Here's the drawing with two shaded views (mm, measured from the low corner). I have some questions. Coordinates: 2 decimals unless noted, no trailing zeros. Loops run counter-clockwise (first coordinate to the right, second up) from the corner with the lowest first, then second, coordinate; pieces in that order, holes last.
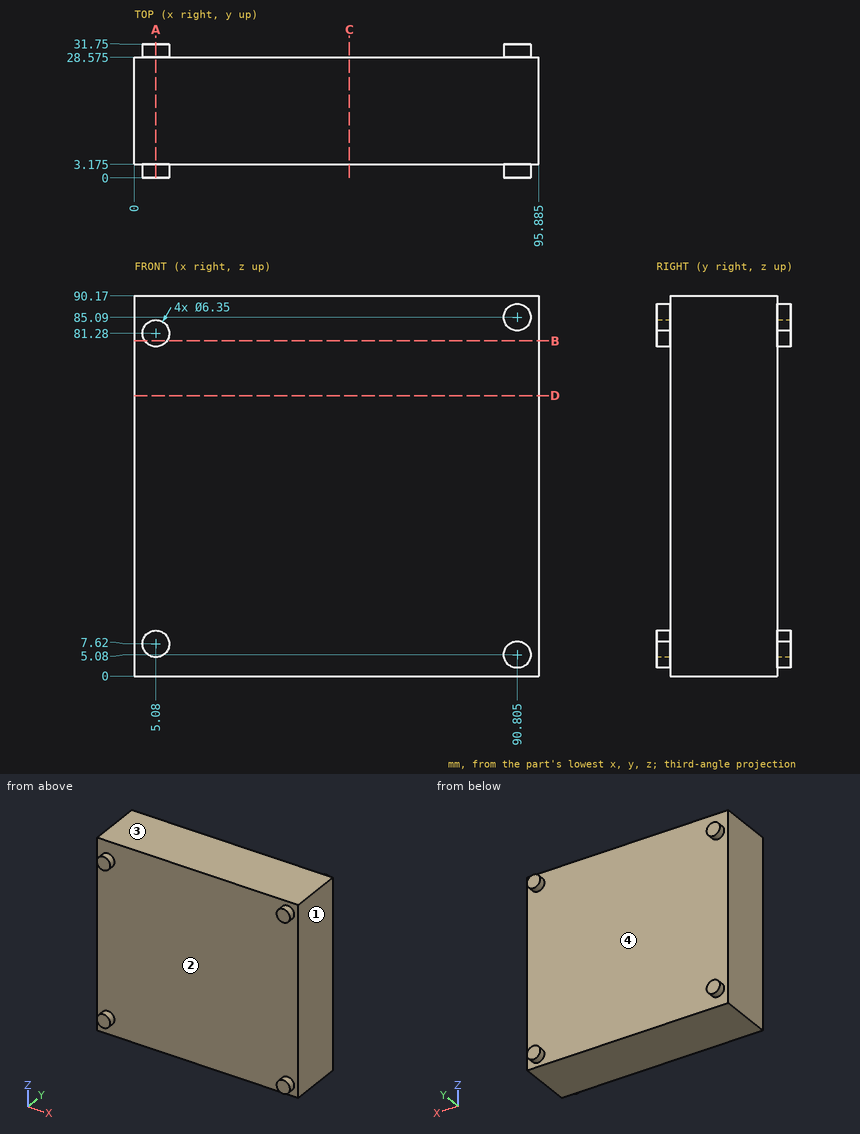
Q1. Please list where this line runs through material, in increasing order: probe 1 along Y at (x, z) = (48.5, 82) (3 decimals).
Q2. Suppose I cut it at C-C on x = 51. Write out the boundary of the cut face in (y, z) (3 decimals).
Q3. Suppose I cut it at B-B on z = 79.5. Write out the boundary of the cut face in (x, y) (3 decimals).
Q4. We'd pull the mould along Z, two halves only. Please class the marked faces 1, 2, 3 and 4: pulls with the +Z half, pulls with the -Z half, needs draft (parallel to the pull), parting line crosses it, or undercut.
Q5. Will these pins go through, and if not, where does the flat tip stop? P1, Ø12, axis at x = 71, z = 26, coming from the +Y side (3 decimals); P2, Ø2, axis at x = 85, y = 22.5, coming from the -Z side; P3, Ø4, axis at x = 30, z = 12, coming from the -Y side (3 decimals).
Q6. Suppose I cut it at A-A on x = 5.08. Write out the boundary of the cut face in (y, z) (3 decimals), and give its area (3 significant figures).
Q7. Suppose I cut it at D-D on z = 66.5. Write out the boundary of the cut face in (x, y) (3 decimals), and give its area (3 significant figures).
Check values:
1. probe 1: y = 3.175 to 28.575
2. outline: (3.175, 0) - (28.575, 0) - (28.575, 90.17) - (3.175, 90.17) - close
3. outline: (0, 3.175) - (2.451, 3.175) - (2.451, 0) - (7.709, 0) - (7.709, 3.175) - (95.885, 3.175) - (95.885, 28.575) - (7.709, 28.575) - (7.709, 31.75) - (2.451, 31.75) - (2.451, 28.575) - (0, 28.575) - close
4. face 1: needs draft
4. face 2: undercut
4. face 3: pulls with the +Z half
4. face 4: undercut
5. P1: stops at y = 28.575
5. P2: stops at z = 0
5. P3: stops at y = 3.175
6. outline: (0, 4.445) - (3.175, 4.445) - (3.175, 0) - (28.575, 0) - (28.575, 4.445) - (31.75, 4.445) - (31.75, 10.795) - (28.575, 10.795) - (28.575, 78.105) - (31.75, 78.105) - (31.75, 84.455) - (28.575, 84.455) - (28.575, 90.17) - (3.175, 90.17) - (3.175, 84.455) - (0, 84.455) - (0, 78.105) - (3.175, 78.105) - (3.175, 10.795) - (0, 10.795) - close
6. area: 2,370 mm2
7. outline: (0, 3.175) - (95.885, 3.175) - (95.885, 28.575) - (0, 28.575) - close
7. area: 2,440 mm2
